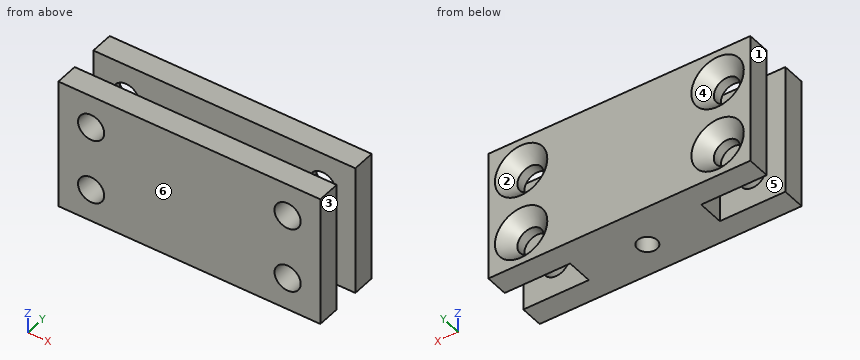
from build123d import *

# Parameters (mm, degrees)
SKETCH_1_R          = 1.5
EXTRUDE_1_DEPTH     = 5
SKETCH_3_W          = 40
SKETCH_3_H          = 3.5
EXTRUDE_2_DEPTH     = 10
SKETCH_2_R          = 2
CUT_EXTRUDE_1_DEPTH = 28.313000567
CHAMFER_1_SIZE      = 2


with BuildPart() as part:
    # 草图1 → 凸台-拉伸1 (new, symmetric)
    with BuildSketch(Plane.XY):
        Polygon((20, 11), (-20, 11), (-20, 7.5), (-10, 7.5), (-10, 3.5), (-20, 3.5), (-20, 0), (0, 0), (20, 0), (20, 3.5), (10, 3.5), (10, 7.5), (20, 7.5), align=None)
        with Locations((0, 5)):
            Circle(SKETCH_1_R, mode=Mode.SUBTRACT)
    extrude(amount=EXTRUDE_1_DEPTH, both=True)

    # 草图3 → 凸台-拉伸2 (add)
    with BuildSketch(Plane.XY.offset(5)):
        with Locations((0, 9.25)):
            Rectangle(SKETCH_3_W, SKETCH_3_H)
        with Locations((0, 1.75)):
            Rectangle(SKETCH_3_W, SKETCH_3_H)
    extrude(amount=EXTRUDE_2_DEPTH)

    # 草图2 → 切除-拉伸1 (cut, through all)
    with BuildSketch(Plane(origin=(0, 0, 0), x_dir=(1, 0, 0), z_dir=(0, 1, 0))):
        with Locations(Location((-15, 0, 0), (0, 0, 270))):
            Circle(SKETCH_2_R)
        with Locations(Location((15, 0, 0), (0, 0, 90))):
            Circle(SKETCH_2_R)
        with Locations(Location((-15, -10, 0), (0, 0, 270))):
            Circle(SKETCH_2_R)
        with Locations(Location((15, -10, 0), (0, 0, 90))):
            Circle(SKETCH_2_R)
    extrude(amount=CUT_EXTRUDE_1_DEPTH, mode=Mode.SUBTRACT)

    # 倒角1
    chamfer_1_edges = [part.edges().sort_by_distance(p)[0] for p in [
        (15, 11, 2),
        (-15, 11, 8),
        (15, 11, 12),
        (-15, 11, -2),
    ]]
    chamfer(chamfer_1_edges, length=CHAMFER_1_SIZE)


solid = part.part
Read the model definition and answer for the solid it produces. Units are mm, in the model's axes. Face numbers are marked on the shaded views. A direction names the side the tool comes from. Coordinates: 2 decimals unless noted, no trailing zeros. Order: outer loops, then holes, each group sorted by start corner. A loop starts at its lowest first (then second) coordinate and runs counter-clockwise, first axis right, second up. Notation, with made-up numbers: M 63,-17 L 110,-17 A18 cw 110,10 Z; hole C -3,57 d4. An arc over 180 degrees is marked long. Put each result on its own line as item: value. Start each with the question number.
Item 1: Section A-A, the plane x = -15 is taken. Determine the outline of the cut face in (y, z), plus the area to 3 significant figures.
Item 2: Section B-B, the plane z = 10 is taken. Determine the outline of the cut face in (x, y), plus the area to 3 significant figures.
Item 3: Section D-D, the plane x = 0.5 is taken. Determine the outline of the cut face in (y, z), plus the area to 3 significant figures.
Item 4: Given pin 1 Ø1.2 at (y, z) = (5.5, 1.5) entering from -X; pin 2 Ø1.5 at (x, z) = (15, 12) entering from +Y; pin 3 Ø3 at (y, z) = (5.5, 0.5) entering from +X, each flat-ended and moving along its own axis, determine where each tip first touches the part or whether it passes through.
Item 5: The mould has two halves that part along X. Classify the marked faces 1, 2, 3 and 4: +X half, -X half, draft (parallel to the pull), parting line (faces both ways), or undercut.
Item 6: Consider probe 1 along Z at (x, y) = (-15, 0.8); probe 2 along X at (y, z) = (7.95, 0); probe 3 along X at (y, z) = (5, 2). Determine where each line is inside the solid, lowest interval first. Write a range as [from, to].
Item 7: For the marked faces 5 and 6, determine the directions among +Z, -Z, +X, -X, +Y, -Y from which every point of the face is accessible in a straight line to the end or side of a thin tool.
Item 8: Section C-C, the plane y = 0.75 is taken. Determine the outline of the cut face in (x, z), plus the area to 3 significant figures.
Computed:
1. outline: M 0,-5 L 3.5,-5 L 3.5,-2 L 0,-2 Z; M 0,2 L 3.5,2 L 3.5,8 L 0,8 Z; M 0,12 L 3.5,12 L 3.5,15 L 0,15 Z; M 7.5,-5 L 11,-5 L 11,-4 L 9,-2 L 7.5,-2 Z; M 7.5,2 L 9,2 L 11,4 L 11,6 L 9,8 L 7.5,8 Z; M 7.5,12 L 9,12 L 11,14 L 11,15 L 7.5,15 Z
1. area: 76.0 mm2
2. outline: M -20,0 L -17,0 L -17,3.5 L -20,3.5 Z; M -20,7.5 L -17,7.5 L -17,9 L -19,11 L -20,11 Z; M -13,0 L 13,0 L 13,3.5 L -13,3.5 Z; M -13,7.5 L 13,7.5 L 13,9 L 11,11 L -11,11 L -13,9 Z; M 17,0 L 20,0 L 20,3.5 L 17,3.5 Z; M 17,7.5 L 20,7.5 L 20,11 L 19,11 L 17,9 Z
2. area: 216 mm2
3. outline: M 0,-5 L 3.59,-5 L 3.59,5 L 3.5,5 L 3.5,15 L 0,15 Z; M 6.41,-5 L 11,-5 L 11,15 L 7.5,15 L 7.5,5 L 6.41,5 Z
3. area: 152 mm2
4. pin 1: stops at x = -10
4. pin 2: stops at y = 9.75
4. pin 3: stops at x = 10
5. face 1: -X half
5. face 2: undercut
5. face 3: +X half
5. face 4: undercut
6. probe 1: z = [-5, -2], [2, 8], [12, 15]
6. probe 2: x = [-20, -17], [-13, 13], [17, 20]
6. probe 3: x = [-10, -1.5], [1.5, 10]
7. face 5: +Z
7. face 6: +Z, -Z, +X, -X, -Y
8. outline: M -20,-5 L 20,-5 L 20,15 L -20,15 Z; hole C -15,0 d4; hole C -15,10 d4; hole C 15,0 d4; hole C 15,10 d4
8. area: 750 mm2
